Verification items for the finished model (mm, model axes). Round coordinates to 2 decimals unless told otherwise and drop trailing zeros. Write each loop counter-clockwise with the first axis right and the second up, starting at its lowest first coordinate (ties: lowest second). Pieces come first, ordered by that corner, then holes.
from build123d import *

# Parameters (mm, degrees)
SKETCH1_W           = 88
SKETCH1_H           = 45
BOSS_EXTRUDE1_DEPTH = 8
SKETCH2_R           = 1.5
CUT_EXTRUDE1_DEPTH  = 144


with BuildPart() as part:
    # Sketch1 → Boss-Extrude1 (new body)
    with BuildSketch(Plane.XY):
        with Locations((44, 22.5)):
            Rectangle(SKETCH1_W, SKETCH1_H)
    extrude(amount=BOSS_EXTRUDE1_DEPTH)

    # Sketch2 → Cut-Extrude1 (cut)
    with BuildSketch(Plane.ZY):
        with Locations((4, 41)):
            Circle(SKETCH2_R)
        with Locations((4, 4)):
            Circle(SKETCH2_R)
    extrude(amount=-CUT_EXTRUDE1_DEPTH, mode=Mode.SUBTRACT)


solid = part.part
Q1. Sectioned sample at C-C (x = 61). Enter the section's corners in (y, z), plus the area to 3 significant figures.
Recorded:
outline: (0, 0) - (45, 0) - (45, 8) - (0, 8) - close; hole circle Ø3 at (4, 4); hole circle Ø3 at (41, 4)
area: 346 mm2
Q2. Release check for a two-part mould opening along Z. For faces 1 (the flat face through (0, 22, 4)), 2 (the cylindrical face through (43.38, 39.67, 4.69)), 3 (the flat face through (43, 23, 8)) record: released by +Z, released by -Z, zero draft, split by the parting line, or undercut.
Recorded:
face 1: zero draft
face 2: undercut
face 3: released by +Z
Q3. Sectioned sample at A-A (y = 4). Enter the section's corners in (x, z), plus the area to 3 significant figures.
Recorded:
outline: (0, 0) - (88, 0) - (88, 2.5) - (0, 2.5) - close; (0, 5.5) - (88, 5.5) - (88, 8) - (0, 8) - close
area: 440 mm2
Q4. Sectioned sample at B-B (z = 4). Enter the section's corners in (x, y), plus the area to 3 significant figures.
Recorded:
outline: (0, 0) - (88, 0) - (88, 2.5) - (0, 2.5) - close; (0, 5.5) - (88, 5.5) - (88, 39.5) - (0, 39.5) - close; (0, 42.5) - (88, 42.5) - (88, 45) - (0, 45) - close
area: 3,430 mm2
Q5. Material ranges on line 1 along Y through (x, z) = (50, 4); line 2 along Y through (x, z) = (45.5, 3); line 3 along Z through (x, y) = (9, 3), recorded low to high.
Recorded:
line 1: y = 0 to 2.5, 5.5 to 39.5, 42.5 to 45
line 2: y = 0 to 2.88, 5.12 to 39.88, 42.12 to 45
line 3: z = 0 to 2.88, 5.12 to 8
